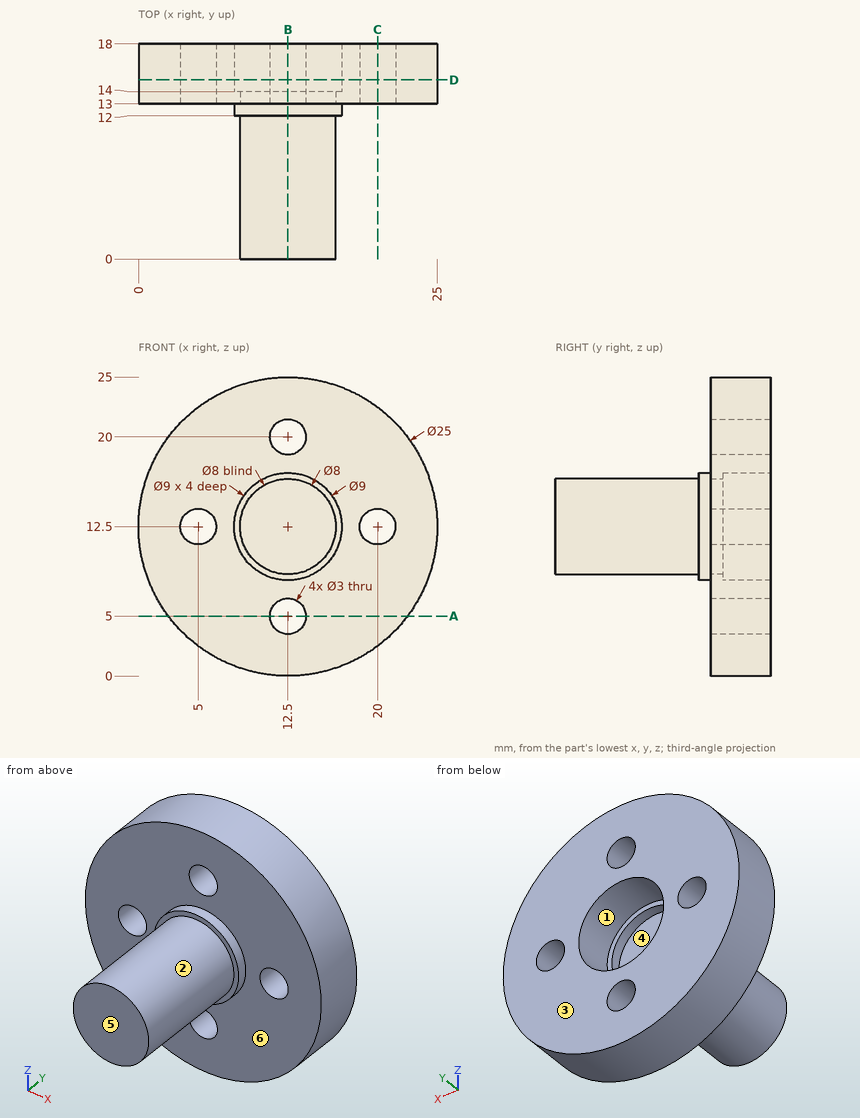
Input: dimensioned drawing with shaded views. Units: mm. Origin: part minimum x, y, z. A direction names the side the tool comes from. Round coordinates to 2 decimals unless told otherwise and drop trailing zeros. Order: outer loops, then holes, each group sorted by start corner. A loop starts at its lowest first (then second) coordinate and runs counter-clockwise, first axis right, second up.
Q1. Mould query, pull axis X, two halves, no side actions, for the marked faces 1, 2 and 3. Classes: released by +X, released by -X, zero draft, split by the parting line, or undercut.
Result sheet:
face 1: undercut
face 2: split by the parting line
face 3: zero draft
Q2. Pin query (flat end, axial travel): pin 1 (8 mm diameter, centred on x = 12.5, z = 12.5, fed in from -Y); pin 2 (10 mm diameter, centred on x = 19.5, y = 14.5, fed in from +Z); pin 3 (5 mm diameter, centred on x = 12.5, z = 5, fed in from -Y); pin 4 (5 mm diameter, centred on x = 19, y = 15, fed in from +Z). Return the tip coordinate at first contact, or that it passes through.
Result sheet:
pin 1: stops at y = 0
pin 2: stops at z = 24.84
pin 3: stops at y = 13
pin 4: stops at z = 24.34
Q3. Section C-C, the plane x = 20. Output: boundary loops of the cut face in (y, z), and give its area (3 significant figures).
Result sheet:
outline: (13, 2.5) - (18, 2.5) - (18, 11) - (13, 11) - close; (13, 14) - (18, 14) - (18, 22.5) - (13, 22.5) - close
area: 85.0 mm2
Q4. Section D-D, the plane y = 15. Output: boundary loops of the cut face in (x, z).
Result sheet:
outline: circle Ø25 at (12.5, 12.5); hole circle Ø3 at (5, 12.5); hole circle Ø9 at (12.5, 12.5); hole circle Ø3 at (12.5, 5); hole circle Ø3 at (12.5, 20); hole circle Ø3 at (20, 12.5)
Q5. Section A-A, the plane z = 5. Output: boundary loops of the cut face in (x, y), and give its area (3 significant figures).
Result sheet:
outline: (2.5, 13) - (11, 13) - (11, 18) - (2.5, 18) - close; (14, 13) - (22.5, 13) - (22.5, 18) - (14, 18) - close
area: 85.0 mm2
Q6. Access query for the marked faces 4, 5 and 6. Directions: +Z, -Z, +X, -X, +Y, -Y. A direction counts if a zero-diameter tool reaches every point of the face in a straight line with its end or side. Return the directions, or none.
Result sheet:
face 4: +Y
face 5: +Z, -Z, +X, -X, -Y
face 6: -Y
Q7. Section B-B, the plane x = 12.5. Output: boundary loops of the cut face in (y, z), and give its area (3 significant figures).
Result sheet:
outline: (0, 8.5) - (12, 8.5) - (12, 8) - (13, 8) - (13, 6.5) - (18, 6.5) - (18, 8) - (14, 8) - (14, 8.5) - (13, 8.5) - (13, 16.5) - (14, 16.5) - (14, 17) - (18, 17) - (18, 18.5) - (13, 18.5) - (13, 17) - (12, 17) - (12, 16.5) - (0, 16.5) - close; (13, 0) - (18, 0) - (18, 3.5) - (13, 3.5) - close; (13, 21.5) - (18, 21.5) - (18, 25) - (13, 25) - close
area: 156 mm2
Q8. Material intervals for probe 1 along X at (y, z) = (13.35, 12.5); probe 2 along Z at (x, y) = (12.75, 4); probe 3 along Y at (x, z) = (1, 10), sorted ascending.
Result sheet:
probe 1: x = 0 to 3.5, 6.5 to 8.5, 16.5 to 18.5, 21.5 to 25
probe 2: z = 8.51 to 16.49
probe 3: y = 13 to 18
